Geometry check sheet. Reference: the model listing, model coordinates, mm. Face numbers are marked on the shaded views. Coordinates: 2 decimals unless noted, no trailing zeros. Loops run counter-clockwise (first coordinate to the right, second up) from the corner with the lowest first, then second, coordinate; pieces in that order, holes last. Notation, with made-up numbers: (68.5, -6.75) -> (91.5, -6.75) arc R12 ccw to (91.5, 6.25) -> close; hole circle Ø2 at (-18, 36.25). An arc over 180 degrees is marked (long way). Answer as a JSON object with one key per item and string values.
from build123d import *

# Parameters (mm, degrees)
SKETCH1_R           = 2.9
SKETCH1_R_2         = 2.225
BOSS_EXTRUDE1_DEPTH = 3


with BuildPart() as part:
    # Sketch1 → Boss-Extrude1 (new body)
    with BuildSketch(Plane.XZ.offset(3)):
        with BuildLine():
            Line((5.581105, 7.9), (-5.581105, 7.9))
            ThreePointArc((-5.581105, 7.9), (-13.481105, 0), (-5.581105, -7.9))
            Line((-5.581105, -7.9), (5.581105, -7.9))
            ThreePointArc((5.581105, -7.9), (13.481105, 0), (5.581105, 7.9))
        make_face()
        with Locations((-5.581105, 0)):
            Circle(SKETCH1_R, mode=Mode.SUBTRACT)
        with Locations((5.581105, 0)):
            Circle(SKETCH1_R_2, mode=Mode.SUBTRACT)
    extrude(amount=-BOSS_EXTRUDE1_DEPTH)


solid = part.part
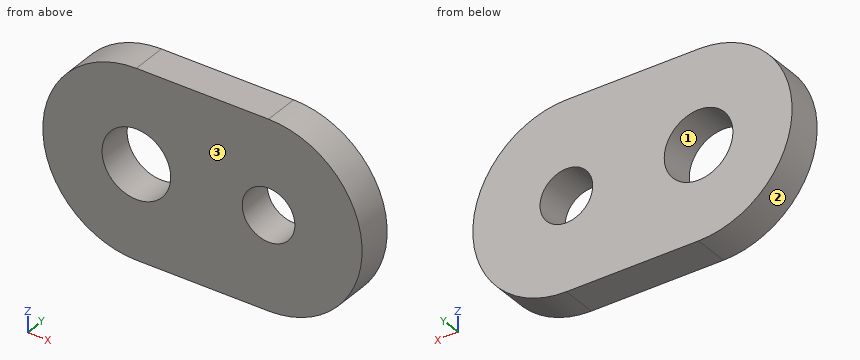
1. Section check A-A, the plane z = 0. Record the boundary of the cut face in (x, y), then the cut area to 3 significant figures.
Evaluation:
{"outline": "(-13.48, -3) -> (-8.48, -3) -> (-8.48, 0) -> (-13.48, 0) -> close; (-2.68, -3) -> (3.36, -3) -> (3.36, 0) -> (-2.68, 0) -> close; (7.81, -3) -> (13.48, -3) -> (13.48, 0) -> (7.81, 0) -> close", "area": "50.1 mm^2"}
2. Section check D-D, the plane x = -4. Record the boundary of the cut face in (y, z).
Evaluation:
{"outline": "(-3, -7.9) -> (0, -7.9) -> (0, -2.43) -> (-3, -2.43) -> close; (-3, 2.43) -> (0, 2.43) -> (0, 7.9) -> (-3, 7.9) -> close"}
3. Section check B-B, the plane x = 4.75. Record the boundary of the cut face in (y, z), then the cut area to 3 significant figures.
Evaluation:
{"outline": "(-3, -7.9) -> (0, -7.9) -> (0, -2.06) -> (-3, -2.06) -> close; (-3, 2.06) -> (0, 2.06) -> (0, 7.9) -> (-3, 7.9) -> close", "area": "35.0 mm^2"}
4. Mould release check, pull along X, two halves, no side actions. Record for the marked faces 1, 2 and 3: released by +X, released by -X, zero draft, split by the parting line, or undercut.
Evaluation:
{"face 1": "undercut", "face 2": "released by -X", "face 3": "zero draft"}
5. Section check C-C, the plane y = -1.4. Record the boundary of the cut face in (x, z) (3 decimals), then the cut area to 3 significant figures.
Evaluation:
{"outline": "(-5.581, -7.9) -> (5.581, -7.9) arc R7.9 ccw to (5.581, 7.9) -> (-5.581, 7.9) arc R7.9 ccw to start; hole circle Ø5.8 at (-5.581, 0); hole circle Ø4.45 at (5.581, 0)", "area": "330 mm^2"}
6. Thickness scan on probe 1 along X at (y, z) = (-2.7, 0.75); probe 2 along X at (y, z) = (-1, 1); probe 3 along Z at (x, y) = (-7.5, -1). Record the ranges inside material, lowest first. Write a range as from..to.
Evaluation:
{"probe 1": "x = -13.45..-8.38, -2.78..3.49, 7.68..13.45", "probe 2": "x = -13.42..-8.3, -2.86..3.59, 7.57..13.42", "probe 3": "z = -7.66..-2.17, 2.17..7.66"}
